```python
from build123d import *

# Parameters (mm, degrees)
SKETCH2_W           = 39.878
SKETCH2_H           = 19.812
BOSS_EXTRUDE1_DEPTH = 40.386
SKETCH3_W           = 19.812
SKETCH3_H           = 5.640095975
BOSS_EXTRUDE2_DEPTH = 7.25
SKETCH4_W           = 19.812
SKETCH4_H           = 5.588
BOSS_EXTRUDE3_DEPTH = 7.25


with BuildPart() as part:
    # Sketch2 → Boss-Extrude1 (new body)
    with BuildSketch(Plane(origin=(0, 0, 0), x_dir=(1, 0, 0), z_dir=(0, 1, 0))):
        with Locations((19.939, 9.906)):
            Rectangle(SKETCH2_W, SKETCH2_H)
    extrude(amount=BOSS_EXTRUDE1_DEPTH)

    # Sketch3 → Boss-Extrude2 (add)
    with BuildSketch(Plane(origin=(39.878, 0, 0), x_dir=(0, 0, -1), z_dir=(1, 0, 0))):
        with Locations((9.906, 30.520047988)):
            Rectangle(SKETCH3_W, SKETCH3_H)
    extrude(amount=BOSS_EXTRUDE2_DEPTH)

    # Sketch4 → Boss-Extrude3 (add)
    with BuildSketch(Plane.ZY):
        with Locations((-9.906, 30.494)):
            Rectangle(SKETCH4_W, SKETCH4_H)
    extrude(amount=BOSS_EXTRUDE3_DEPTH)


solid = part.part
```
Verification items for the finished model (mm, model axes). A direction names the side the tool comes from. Coordinates: 2 decimals unless noted, no trailing zeros. Write each loop counter-clockwise with the first axis right and the second up, starting at its lowest first coordinate (ties: lowest second). Pieces come first, ordered by that corner, then holes. Notation, with made-up numbers: (77, -14) - (121, -14) arc R27 cw to (121, 18) - close; hole circle Ø9 at (10.5, 27). An arc over 180 degrees is marked (long way). Write item = value, one per line.
Q1. Material ranges on L1, parallel to X at y = 36, z = -8; L2, parallel to Y at x = -2, z = -4.25, recorded low to high. Write a range as from..to.
Answer:
L1 = 0..39.88
L2 = 27.7..33.29
Q2. Go/stop test with flat-tipped pins: pin 1 Ø10 at (y, z) = (22, -10.5) entering from +X; pin 2 Ø3 at (y, z) = (21, -7.5) entering from -X; pin 3 Ø6 at (x, z) = (43.5, -10) entering from +Y. Record where each tip stops, or that it passes through.
Answer:
pin_1 = 39.88
pin_2 = 0
pin_3 = 33.34
Q3. Cross-section at B-B (y = 20). Enter the section's corners in (x, z), plus the area to 3 significant figures.
Answer:
outline = (0, -19.81) - (39.88, -19.81) - (39.88, 0) - (0, 0) - close
area = 790 mm²
Q4. Cross-section at C-C (x = 43). Enter the section's corners in (y, z), plus the area to 3 significant figures.
Answer:
outline = (27.7, -19.81) - (33.34, -19.81) - (33.34, 0) - (27.7, 0) - close
area = 112 mm²
Q5. Cross-section at A-A (z = -16.5). Enter the section's corners in (x, y).
Answer:
outline = (-7.25, 27.7) - (0, 27.7) - (0, 0) - (39.88, 0) - (39.88, 27.7) - (47.13, 27.7) - (47.13, 33.34) - (39.88, 33.34) - (39.88, 40.39) - (0, 40.39) - (0, 33.29) - (-7.25, 33.29) - close
Q6. Access from +Z, -Z, +X, -X, +Y, -Y to the whole of each face (thin tool, end or side, straight path). Record for faces 1 (the face through (43, 33.34, -10)), 2 (the face through (43, 27.7, -10)), 3 (the face through (-4, 27.7, -10)).
Answer:
face_1 = +Z, -Z, +X, +Y
face_2 = +Z, -Z, +X, -Y
face_3 = +Z, -Z, -X, -Y
